The drawing under review shows one solid part. Ordinate dimensions are in mm from its lowest x, y, z. A direction names the side the tool comes from. Give positions to 0.01 mm unless a question says otherwise; leave off trailing zeros. Order: outer loops, then holes, each group sorted by start corner. A loop starts at its lowest first (then second) coordinate and runs counter-clockwise, first axis right, second up. Notation, with made-up numbers: (-15.5, 49) -> (41.5, 49) arc R9 ccw to (41.5, 53) -> close; hole circle Ø2 at (18.5, 65.5). An arc over 180 degrees is marked (long way). Return JSON: item names as keys, results as strings. Group by question number.
1) Add section B-B (x = 15). Give the boundary of the cut face in (y, z), then the cut area to 3 significant figures.
2) To check wall thickness, follow line 1 along Z through (x, y) = (15.5, 15); line 2 along Y through (x, z) = (15.5, 77); line 3 along X through (y, z) = (15.25, 21). State the ranges of each line that lie inside material, in increasing order.
3) For the marked faces 1 and 2, list the 3-axis set-ups (+Z, -Z, +X, -X, +Y, -Y) from which the entire face can be reached by the end or side of a thin tool; tool diameter is ignored.
4) Insertion check: P1, Ø12, axis at x = 5.5, y = 25, coming from the +Z side; P2, Ø2, axis at y = 15.5, z = 35.5, coming from the +X side; P3, Ø1.5, axis at y = 23.5, z = 55, coming from the +X side. Each pin has a flat end and moves straight along its axis. Give the tip position at first contact, or say it passes through.
5) Add section D-D (z = 77). Give the boundary of the cut face in (x, y).
6) Add section A-A (y = 15). Give the boundary of the cut face in (x, z).
7) Add section C-C (z = 65). Give the boundary of the cut face in (x, y).
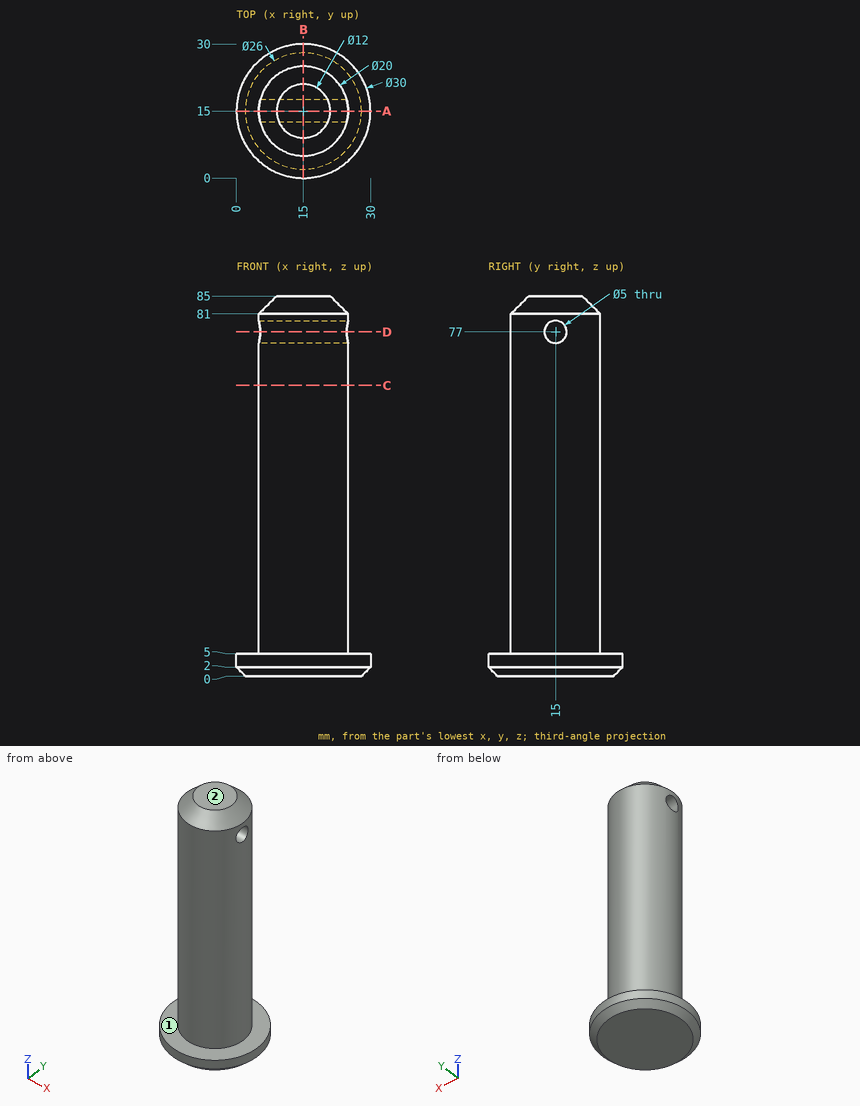
Evaluation:
{
 "1": {"outline": "(0, 2) -> (2, 0) -> (28, 0) -> (30, 2) -> (30, 5) -> (25, 5) -> (25, 81) -> (21, 85) -> (9, 85) -> (5, 81) -> (5, 5) -> (0, 5) -> close; hole circle Ø5 at (15, 77)", "area": "1,710 mm^2"},
 "2": {"line 1": "0 to 74.5, 79.5 to 85", "line 2": "5.01 to 12.5, 17.5 to 24.99", "line 3": "5 to 25"},
 "3": {"face 1": "+Z", "face 2": "+Z, +X, -X, +Y, -Y"},
 "4": {"P1": "z = 83.21", "P2": "x = 25", "P3": "x = 21.32"},
 "5": {"outline": "(5.32, 12.5) arc R10 ccw to (24.68, 12.5) -> close; (5.32, 17.5) -> (24.68, 17.5) arc R10 ccw to start"},
 "6": {"outline": "(0, 2) -> (2, 0) -> (28, 0) -> (30, 2) -> (30, 5) -> (25, 5) -> (25, 74.5) -> (5, 74.5) -> (5, 5) -> (0, 5) -> close; (5, 79.5) -> (25, 79.5) -> (25, 81) -> (21, 85) -> (9, 85) -> (5, 81) -> close"},
 "7": {"outline": "circle Ø20 at (15, 15)"}
}
